Here's the drawing with two shaded views (mm, measured from the low corner). I have some questions. Give positions to 0.01 mm unless a question says otherwise; leave off trailing zeros. Order: outer loops, then holes, each group sorted by start corner. A loop starts at its lowest first (then second) coordinate and runs counter-clockwise, first axis right, second up. Notation, with made-up numbers: (-2, 84) - (21, 84) arc R32 ccw to (21, 114) - close; hole circle Ø6 at (70, 69). An arc over 180 degrees is marked (long way). Use one line per item in the form item = value. Start each with the question number.
1) Suppose I cut it at A-A, the plane x = 35. Write out the boundary of the cut face in (y, z).
2) We'd pull the mould along X, two halves only. Please class the marked faces 1, 2 and 3: released by +X, released by -X, zero draft, split by the parting line, or undercut.
3) Suppose I cut it at B-B, the plane z = 35. Write out the boundary of the cut face in (x, y).
4) For pin 1 (2 mm diameter, centred on x = 63, y = 8.5, fed in from -Z); pin 2 (5 mm diameter, centred on x = 54, y = 5.5, fed in from +Z); pin 3 (1 mm diameter, centred on x = 7, y = 6, fed in from +Z), each with a flat end and sliding along its axis, tell me the tip position at first contact or that it passes through.
5) Suppose I cut it at C-C, the plane z = 42.5. Write out the boundary of the cut face in (x, y) (1 decimal).
6) Suppose I cut it at D-D, the plane x = 43.5. Write out the boundary of the cut face in (y, z).
7) Please list where these lines run through material, in increasing order: probe 1 along Z at (x, y) = (35, 4); probe 2 along X at (y, z) = (0.5, 35).
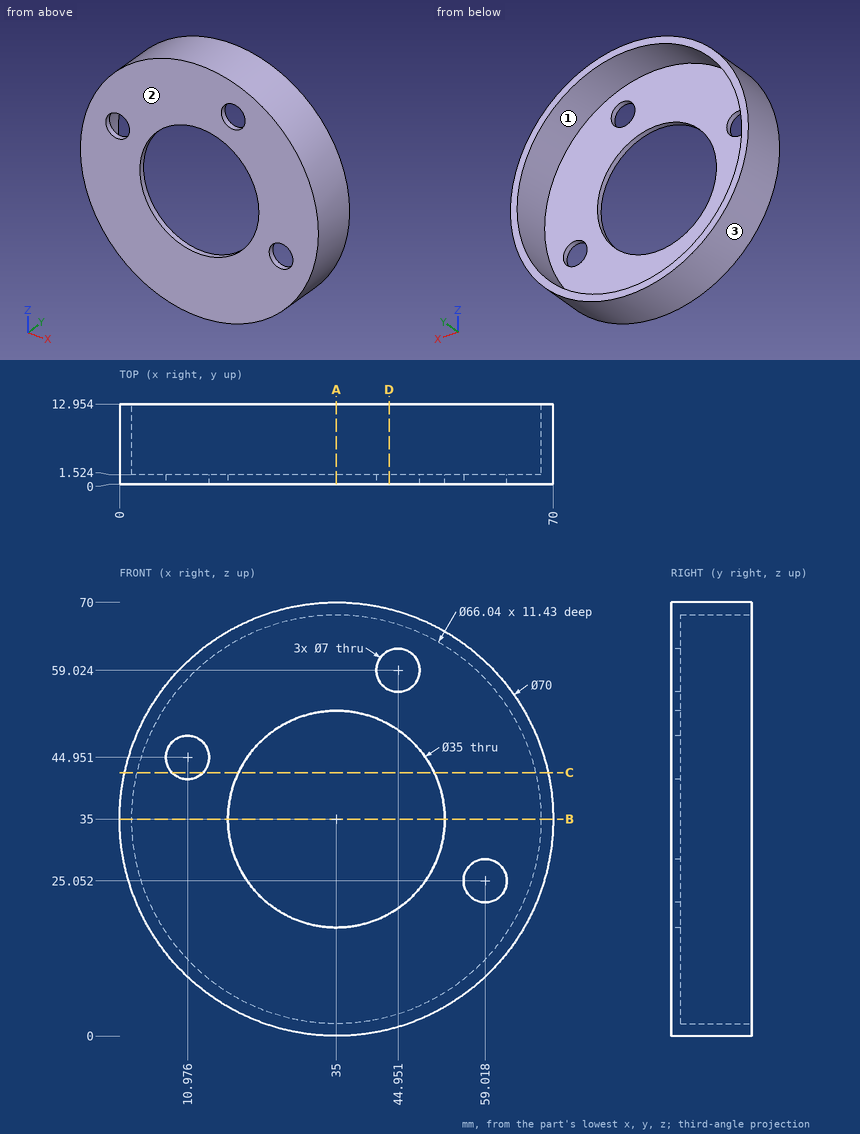
Result sheet:
q1.outline = (0, 0) - (12.95, 0) - (12.95, 1.98) - (1.52, 1.98) - (1.52, 17.5) - (0, 17.5) - close; (0, 52.5) - (1.52, 52.5) - (1.52, 68.02) - (12.95, 68.02) - (12.95, 70) - (0, 70) - close
q2.face_1 = undercut
q2.face_2 = zero draft
q2.face_3 = split by the parting line
q3.outline = (0, 0) - (17.5, 0) - (17.5, 1.52) - (1.98, 1.52) - (1.98, 12.95) - (0, 12.95) - close; (52.5, 0) - (70, 0) - (70, 12.95) - (68.02, 12.95) - (68.02, 1.52) - (52.5, 1.52) - close
q4.pin_1 = 12.73
q4.pin_2 = 65.87
q4.pin_3 = 56.65
q5.outline = (0.8, 0) - (8.5, 0) - (8.5, 1.5) - (2.8, 1.5) - (2.8, 13) - (0.8, 13) - close; (13.5, 0) - (19.2, 0) - (19.2, 1.5) - (13.5, 1.5) - close; (50.8, 0) - (69.2, 0) - (69.2, 13) - (67.2, 13) - (67.2, 1.5) - (50.8, 1.5) - close
q6.outline = (0, 1.05) - (12.95, 1.05) - (12.95, 3.09) - (1.52, 3.09) - (1.52, 19.7) - (0, 19.7) - close; (0, 50.3) - (1.52, 50.3) - (1.52, 55.84) - (0, 55.84) - close; (0, 62.21) - (1.52, 62.21) - (1.52, 66.91) - (12.95, 66.91) - (12.95, 68.95) - (0, 68.95) - close
q7.probe_1 = 0 to 1.98, 68.02 to 70
q7.probe_2 = 0 to 17.5, 52.5 to 70
